Can you work these out from the drawing? Everything is in mm from the part's minimum corner. A direction names the side the tool comes from. Round coordinates to 2 decimals unless told otherwise and drop trailing zeros. Loops run counter-clockwise (first coordinate to the right, second up) from the corner with the lowest first, then second, coordinate; pieces in that order, holes last. Notation, with made-up numbers: M 54,48 L 90,48 A20 ccw 90,69 Z; hole C 22,-2.5 d10. An arc over 180 degrees is marked long. Use a Markdown table: item, result.
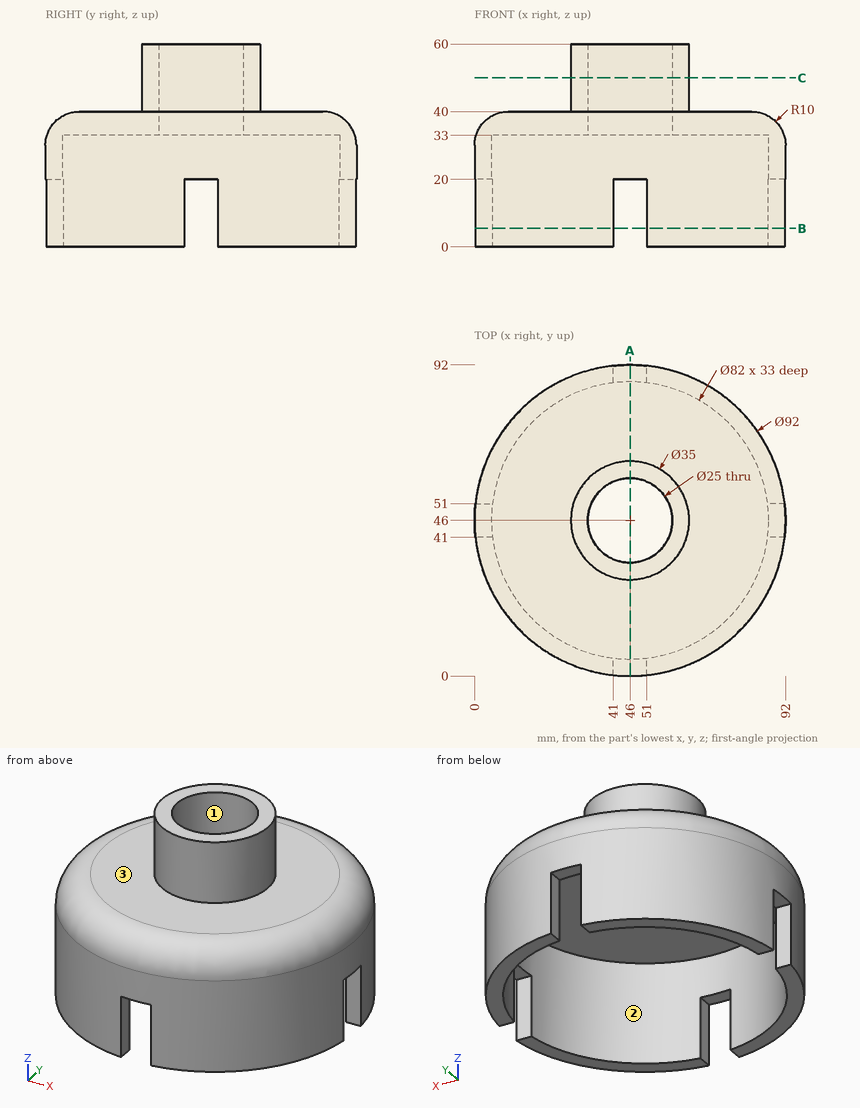
Q1. Imagine slicing it at A-A, the plane x = 46. Please give me the cut outline in (y, z), then the cut area to 3 significant figures.
Return value:
| item | result |
|---|---|
| outline | M 0,20 L 5,20 L 5,33 L 33.5,33 L 33.5,60 L 28.5,60 L 28.5,40 L 10,40 A10 ccw 0,30 Z; M 58.5,33 L 87,33 L 87,20 L 92,20 L 92,30 A10 ccw 82,40 L 63.5,40 L 63.5,60 L 58.5,60 Z |
| area | 756 mm^2 |
Q2. For the marked faces 1, 2 and 3, which set-ups out of +Z, -Z, +X, -X, +Y, -Y let a thin tool reach every point of the face, with its end or its side?
Return value:
| item | result |
|---|---|
| face 1 | +Z, -Z |
| face 2 | -Z |
| face 3 | +Z |
Q3. Imagine slicing it at B-B, the plane z = 5.5. Please give me the cut outline in (x, y).
Return value:
| item | result |
|---|---|
| outline | M 0.27,41 A46 ccw 41,0.27 L 41,5.31 A41 cw 5.31,41 Z; M 0.27,51 L 5.31,51 A41 cw 41,86.69 L 41,91.73 A46 ccw Z; M 51,0.27 A46 ccw 91.73,41 L 86.69,41 A41 cw 51,5.31 Z; M 51,86.69 A41 cw 86.69,51 L 91.73,51 A46 ccw 51,91.73 Z |
Q4. Imagine slicing it at C-C, the plane z = 50. Please give me the cut outline in (x, y).
Return value:
| item | result |
|---|---|
| outline | C 46,46 d35; hole C 46,46 d25 |
Q5. Will these pins go through, and if not, where does the flat tip stop? P1, Ø1.5, axis at y = 88.5, z = 15, coming from the +X side; P2, Ø2.5, axis at x = 4, z = 12.5, coming from the +Y side; P3, Ø10, axis at x = 16, y = 59.5, coming from the -Z side.
Return value:
| item | result |
|---|---|
| P1 | stops at x = 65.31 |
| P2 | stops at y = 67.34 |
| P3 | stops at z = 33 |
Q6. I need wall thicknesses on line 1 (Y direction, x = 41, z = 26); line 2 (Y direction, x = 46, z = 23); line 3 (X direction, y = 45, z = 27). Which ranges of each line are inside material? Lowest first, please. Write a range as from..to.
Return value:
| item | result |
|---|---|
| line 1 | y = 0.27..5.31, 86.69..91.73 |
| line 2 | y = 0..5, 87..92 |
| line 3 | x = 0.01..5.01, 86.99..91.99 |
